Check sheet for the modelled part. Datum: model origin and axes. Units: mm. Face numbers are marked on the shaded views. A direction names the side the tool comes from. Round coordinates to 2 decimals unless told otherwise and drop trailing zeros. Loops run counter-clockwise (first coordinate to the right, second up) from the corner with the lowest first, then second, coordinate; pieces in that order, holes last. Notation, with made-up numbers: (-22.5, 77.25) - (-13.5, 77.25) arc R18 ccw to (-13.5, 107.25) - close; hole circle Ø9 at (57, 43). An arc over 180 degrees is marked (long way). Return JSON: item names as keys, results as strings.
from build123d import *
from build123d.topology import SkipClean

# Parameters (mm, degrees)
SKETCH1_R           = 76.2
SKETCH1_R_2         = 14.224
BOSS_EXTRUDE1_DEPTH = 3.81
SKETCH3_R           = 38.1
SKETCH3_R_2         = 35.56
BOSS_EXTRUDE3_DEPTH = 7.62
BOSS_EXTRUDE4_DEPTH = 7.62
SKETCH4_R           = 16
SKETCH4_R_2         = 11
BOSS_EXTRUDE5_DEPTH = 7


with BuildPart() as part:
    # Sketch1 → Boss-Extrude1 (new body)
    with BuildSketch(Plane(origin=(0, 0, 0), x_dir=(1, 0, 0), z_dir=(0, 1, 0))):
        with Locations(Location((0, 0, 0), (0, 0, 90))):
            Circle(SKETCH1_R)
        with Locations(Location((-57.15, 0, 0), (0, 0, 90))):
            Circle(SKETCH1_R_2, mode=Mode.SUBTRACT)
        with Locations(Location((-46.235321229, 33.591927169, 0), (0, 0, 90))):
            Circle(SKETCH1_R_2, mode=Mode.SUBTRACT)
        with Locations(Location((-17.660321229, 54.352879906, 0), (0, 0, 90))):
            Circle(SKETCH1_R_2, mode=Mode.SUBTRACT)
        with Locations(Location((17.660321229, 54.352879906, 0), (0, 0, 90))):
            Circle(SKETCH1_R_2, mode=Mode.SUBTRACT)
        with Locations(Location((46.235321229, 33.591927169, 0), (0, 0, 90))):
            Circle(SKETCH1_R_2, mode=Mode.SUBTRACT)
        with Locations(Location((57.15, 0, 0), (0, 0, 90))):
            Circle(SKETCH1_R_2, mode=Mode.SUBTRACT)
        with Locations(Location((46.235321229, -33.591927169, 0), (0, 0, 90))):
            Circle(SKETCH1_R_2, mode=Mode.SUBTRACT)
        with Locations(Location((17.660321229, -54.352879906, 0), (0, 0, 90))):
            Circle(SKETCH1_R_2, mode=Mode.SUBTRACT)
        with Locations(Location((-17.660321229, -54.352879906, 0), (0, 0, 90))):
            Circle(SKETCH1_R_2, mode=Mode.SUBTRACT)
        with Locations(Location((-46.235321229, -33.591927169, 0), (0, 0, 90))):
            Circle(SKETCH1_R_2, mode=Mode.SUBTRACT)
    extrude(amount=BOSS_EXTRUDE1_DEPTH)

    # Sketch3 → Boss-Extrude3 (add)
    with BuildSketch(Plane(origin=(0, 3.81, 0), x_dir=(1, 0, 0), z_dir=(0, 1, 0))):
        with Locations(Location((0, 0, 0), (0, 0, 90))):
            Circle(SKETCH3_R)
        with Locations(Location((0, 0, 0), (0, 0, 90))):
            Circle(SKETCH3_R_2, mode=Mode.SUBTRACT)
    extrude(amount=BOSS_EXTRUDE3_DEPTH)

    # Sketch2 → Boss-Extrude4 (add)
    with SkipClean():  # the faces are left unmerged after this step: merging them gives an invalid solid
        with BuildSketch(Plane(origin=(0, 3.81, 0), x_dir=(1, 0, 0), z_dir=(0, 1, 0))):
            with BuildLine():
                Line((-72.852892077, -22.335982539), (-36.607568562, -10.559163032))
                ThreePointArc((-36.607568562, -10.559163032), (-36.235253271, -11.773547486), (-35.822665397, -12.974846584))
                Line((-35.822665397, -12.974846584), (-72.067988912, -24.75166609))
                ThreePointArc((-72.067988912, -24.75166609), (-72.470506542, -23.547094971), (-72.852892077, -22.335982539))
            make_face()
            with BuildLine():
                Line((-72.067988912, 24.75166609), (-35.822665397, 12.974846584))
                ThreePointArc((-35.822665397, 12.974846584), (-36.235253271, 11.773547486), (-36.607568562, 10.559163032))
                Line((-36.607568562, 10.559163032), (-72.852892077, 22.335982539))
                ThreePointArc((-72.852892077, 22.335982539), (-72.470506542, 23.547094971), (-72.067988912, 24.75166609))
            make_face()
            with BuildLine():
                Line((-43.755563483, 62.385019551), (-21.354721617, 31.552905804))
                ThreePointArc((-21.354721617, 31.552905804), (-22.394618112, 30.823547486), (-23.409624783, 30.059931263))
                Line((-23.409624783, 30.059931263), (-45.810466648, 60.89204501))
                ThreePointArc((-45.810466648, 60.89204501), (-44.789236225, 61.647094971), (-43.755563483, 62.385019551))
            make_face()
            with BuildLine():
                Line((1.27, 76.189415932), (1.27, 38.07882745))
                ThreePointArc((1.27, 38.07882745), (0, 38.1), (-1.27, 38.07882745))
                Line((-1.27, 38.07882745), (-1.27, 76.189415932))
                ThreePointArc((-1.27, 76.189415932), (0, 76.2), (1.27, 76.189415932))
            make_face()
            with BuildLine():
                Line((45.810466648, 60.89204501), (23.409624783, 30.059931263))
                ThreePointArc((23.409624783, 30.059931263), (22.394618112, 30.823547486), (21.354721617, 31.552905804))
                Line((21.354721617, 31.552905804), (43.755563483, 62.385019551))
                ThreePointArc((43.755563483, 62.385019551), (44.789236225, 61.647094971), (45.810466648, 60.89204501))
            make_face()
            with BuildLine():
                Line((72.852892077, 22.335982539), (36.607568562, 10.559163032))
                ThreePointArc((36.607568562, 10.559163032), (36.235253271, 11.773547486), (35.822665397, 12.974846584))
                Line((35.822665397, 12.974846584), (72.067988912, 24.75166609))
                ThreePointArc((72.067988912, 24.75166609), (72.470506542, 23.547094971), (72.852892077, 22.335982539))
            make_face()
            with BuildLine():
                Line((72.067988912, -24.75166609), (35.822665397, -12.974846584))
                ThreePointArc((35.822665397, -12.974846584), (36.235253271, -11.773547486), (36.607568562, -10.559163032))
                Line((36.607568562, -10.559163032), (72.852892077, -22.335982539))
                ThreePointArc((72.852892077, -22.335982539), (72.470506542, -23.547094971), (72.067988912, -24.75166609))
            make_face()
            with BuildLine():
                Line((43.755563483, -62.385019551), (21.354721617, -31.552905804))
                ThreePointArc((21.354721617, -31.552905804), (22.394618112, -30.823547486), (23.409624783, -30.059931263))
                Line((23.409624783, -30.059931263), (45.810466648, -60.89204501))
                ThreePointArc((45.810466648, -60.89204501), (44.789236225, -61.647094971), (43.755563483, -62.385019551))
            make_face()
            with BuildLine():
                Line((-1.27, -76.189415932), (-1.27, -38.07882745))
                ThreePointArc((-1.27, -38.07882745), (0, -38.1), (1.27, -38.07882745))
                Line((1.27, -38.07882745), (1.27, -76.189415932))
                ThreePointArc((1.27, -76.189415932), (0, -76.2), (-1.27, -76.189415932))
            make_face()
            with BuildLine():
                Line((-45.810466648, -60.89204501), (-23.409624783, -30.059931263))
                ThreePointArc((-23.409624783, -30.059931263), (-22.394618112, -30.823547486), (-21.354721617, -31.552905804))
                Line((-21.354721617, -31.552905804), (-43.755563483, -62.385019551))
                ThreePointArc((-43.755563483, -62.385019551), (-44.789236225, -61.647094971), (-45.810466648, -60.89204501))
            make_face()
        extrude(amount=BOSS_EXTRUDE4_DEPTH)

    # Sketch4 → Boss-Extrude5 (add)
    with SkipClean():  # the faces are left unmerged after this step: merging them gives an invalid solid
        with BuildSketch(Plane(origin=(0, 3.81, 0), x_dir=(1, 0, 0), z_dir=(0, 1, 0))):
            with Locations(Location((0, 0, 0), (0, 0, 270))):
                Circle(SKETCH4_R)
            with Locations(Location((0, 0, 0), (0, 0, 270))):
                Circle(SKETCH4_R_2, mode=Mode.SUBTRACT)
        extrude(amount=BOSS_EXTRUDE5_DEPTH)


solid = part.part
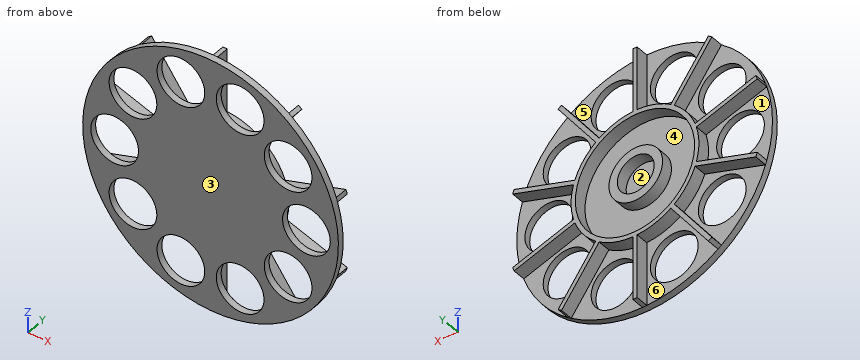
Q1. Depth check by flat-ended pin: P1, Ø14.5, axis at x = -49, z = -37.5, coming from the +Y side; P2, Ø2.5, axis at y = 7.5, z = -61, coming from the -X side; P3, Ø4, axis at y = 9.5, z = 49.5, coming from the -X side; P4, Ø5, axis at x = -29, z = 47.5, coming from the +Y side. Enter the tip coordinate at first touch or a pass-through.
Answer key:
{"P1": "passes through", "P2": "stops at x = -45.81", "P3": "stops at x = -38.99", "P4": "stops at y = 3.81"}
Q2. Sectioned sample at B-B (y = 6). State how many separate pieces and enclosed holes the cut face has, plus the area to 3 significant figures.
Answer key:
{"separate pieces": "2", "enclosed holes": "2", "area": "1,980 mm²"}
Q3. Sectioned sample at D-D (z = 52.5). Enter the section's corners in (x, y).
Answer key:
{"outline": "(-55.23, 0) - (-31.76, 0) - (-31.76, 3.81) - (-36.57, 3.81) - (-36.57, 11.43) - (-39.71, 11.43) - (-39.71, 3.81) - (-55.23, 3.81) - close; (-3.56, 0) - (3.56, 0) - (3.56, 3.81) - (1.27, 3.81) - (1.27, 11.43) - (-1.27, 11.43) - (-1.27, 3.81) - (-3.56, 3.81) - close; (31.76, 0) - (55.23, 0) - (55.23, 3.81) - (39.71, 3.81) - (39.71, 11.43) - (36.57, 11.43) - (36.57, 3.81) - (31.76, 3.81) - close"}
Q4. Draft check along Z on the marked faces 1, 2 and 3. Enter one of: released by +Z, released by -Z, zero draft, split by the parting line, or undercut.
Answer key:
{"face 1": "undercut", "face 2": "undercut", "face 3": "zero draft"}
Q5. Sectioned sample at C-C (z = 33.5). Enter the section's corners in (x, y).
Answer key:
{"outline": "(-68.44, 0) - (-60.46, 0) - (-60.46, 3.81) - (-68.44, 3.81) - close; (-32.01, 0) - (32.01, 0) - (32.01, 3.81) - (25.91, 3.81) - (25.91, 11.43) - (22.77, 11.43) - (22.77, 3.81) - (18.15, 3.81) - (18.15, 11.43) - (11.93, 11.43) - (11.93, 3.81) - (-11.93, 3.81) - (-11.93, 11.43) - (-18.15, 11.43) - (-18.15, 3.81) - (-22.77, 3.81) - (-22.77, 11.43) - (-25.91, 11.43) - (-25.91, 3.81) - (-32.01, 3.81) - close; (60.46, 0) - (68.44, 0) - (68.44, 3.81) - (60.46, 3.81) - close"}
Q6. Scan lines: probe 1 along X at (y, z) = (9, 0); probe 2 along Z at (x, y) = (-57.15, 2.4); probe 3 along Z at (x, y) = (-14.5, 4.5). Record each from-to range of solid material in increasing order. Write a range as [from, to].
Answer key:
{"probe 1": "x = [-38.1, -35.56], [-16, -11], [11, 16], [35.56, 38.1]", "probe 2": "z = [-50.4, -42.71], [-24.47, -14.22], [14.22, 24.47], [42.71, 50.4]", "probe 3": "z = [-35.23, -32.47], [-6.76, 6.76], [32.47, 35.23]"}
Q7. Tool access check on the marked faces 4, 5 and 6. Record the directions out of +Z, -Z, +X, -X, +Y, -Y that give a thin tool (end or side, any length) a straight path to the whole face; none if there is none.
Answer key:
{"face 4": "+Y", "face 5": "+Z, +Y", "face 6": "-Z, +Y"}
Q8. Sectioned sample at A-A (z = 0). Enter the section's corners in (x, y).
Answer key:
{"outline": "(-76.2, 0) - (-71.37, 0) - (-71.37, 3.81) - (-76.2, 3.81) - close; (-42.93, 0) - (42.93, 0) - (42.93, 3.81) - (38.1, 3.81) - (38.1, 11.43) - (35.56, 11.43) - (35.56, 3.81) - (16, 3.81) - (16, 10.81) - (11, 10.81) - (11, 3.81) - (-11, 3.81) - (-11, 10.81) - (-16, 10.81) - (-16, 3.81) - (-35.56, 3.81) - (-35.56, 11.43) - (-38.1, 11.43) - (-38.1, 3.81) - (-42.93, 3.81) - close; (71.37, 0) - (76.2, 0) - (76.2, 3.81) - (71.37, 3.81) - close"}
